Can you work these out from the model? Positions are in its coordinate system, mm. A direction names the side the tool comes from. Give positions to 0.01 mm unless a question says otherwise; leave off trailing zeros. Order: outer loops, then holes, each group sorted by start corner. A loop starts at its lowest first (then second) coordinate and runs counter-clockwise, first axis right, second up. Notation, with made-up numbers: M -7,-36.75 L 7,-36.75 A21 cw 7,-2.75 Z; hole C -2.5,-15 d3. An arc over 180 degrees is marked long. Write each question's results on one line, items separated by ' | '.
from build123d import *

# Parameters (mm, degrees)
SKETCH_1_R          = 10
EXTRUDE_1_DEPTH     = 20
SKETCH_2_R          = 5
EXTRUDE_2_DEPTH     = 5
SKETCH_4_R          = 5.5
SKETCH_4_R_2        = 5
EXTRUDE_3_DEPTH     = 1
SKETCH_5_R          = 1.65
CUT_EXTRUDE_1_DEPTH = 10
SKETCH_6_R          = 5
EXTRUDE_4_DEPTH     = 35.5
SKETCH_7_OUTSIDE_W  = 35.358
SKETCH_7_OUTSIDE_H  = 35.358
SKETCH_7_OUTSIDE_R  = 4
CUT_EXTRUDE_2_DEPTH = 16
SKETCH_8_R          = 1.65
CUT_EXTRUDE_3_DEPTH = 10
SKETCH_9_R          = 4
CUT_EXTRUDE_4_DEPTH = 0.8


with BuildPart() as part:
    # ｽｹｯﾁ1 → ﾎﾞｽ - 押し出し1 (new body)
    with BuildSketch(Plane.XY):
        Circle(SKETCH_1_R)
    extrude(amount=EXTRUDE_1_DEPTH)

    # ｽｹｯﾁ2 → ﾎﾞｽ - 押し出し2 (add)
    with BuildSketch(Plane.XY.offset(20)):
        Circle(SKETCH_2_R)
    extrude(amount=EXTRUDE_2_DEPTH)

    # ｽｹｯﾁ4 → ﾎﾞｽ - 押し出し3 (add)
    with BuildSketch(Plane.XY.offset(20)):
        Circle(SKETCH_4_R)
        Circle(SKETCH_4_R_2, mode=Mode.SUBTRACT)
    extrude(amount=EXTRUDE_3_DEPTH)

    # ｽｹｯﾁ5 → ｶｯﾄ - 押し出し1 (cut)
    with BuildSketch(Plane(origin=(0, 0, 0), x_dir=(-1, 0, 0), z_dir=(0, 0, -1))):
        with Locations((0, 6)):
            Circle(SKETCH_5_R)
        with Locations(Location((0, -6, 0), (0, 0, 180))):
            Circle(SKETCH_5_R)
    extrude(amount=-CUT_EXTRUDE_1_DEPTH, mode=Mode.SUBTRACT)

    # ｽｹｯﾁ6 → ﾎﾞｽ - 押し出し4 (add)
    with BuildSketch(Plane.XY.offset(25)):
        Circle(SKETCH_6_R)
    extrude(amount=EXTRUDE_4_DEPTH)

    # ｽｹｯﾁ7 outside → ｶｯﾄ - 押し出し2 (cut)
    with BuildSketch(Plane.XY.offset(60.5)):
        Rectangle(SKETCH_7_OUTSIDE_W, SKETCH_7_OUTSIDE_H)
        Circle(SKETCH_7_OUTSIDE_R, mode=Mode.SUBTRACT)
    extrude(amount=-CUT_EXTRUDE_2_DEPTH, mode=Mode.SUBTRACT)

    # ｽｹｯﾁ8 → ｶｯﾄ - 押し出し3 (cut)
    with BuildSketch(Plane.XY.offset(60.5)):
        Circle(SKETCH_8_R)
    extrude(amount=-CUT_EXTRUDE_3_DEPTH, mode=Mode.SUBTRACT)

    # ｽｹｯﾁ9 → ｶｯﾄ - 押し出し4 (cut)
    with BuildSketch(Plane.XY.offset(60.5)):
        Circle(SKETCH_9_R)
    extrude(amount=-CUT_EXTRUDE_4_DEPTH, mode=Mode.SUBTRACT)


solid = part.part
(1) Imagine slicing it at B-B, the plane y = 0. Write out the boundary of the cut face in (x, z).
Data:
outline: M -10,0 L 10,0 L 10,20 L 5.5,20 L 5.5,21 L 5,21 L 5,44.5 L 4,44.5 L 4,59.7 L 1.65,59.7 L 1.65,50.5 L -1.65,50.5 L -1.65,59.7 L -4,59.7 L -4,44.5 L -5,44.5 L -5,21 L -5.5,21 L -5.5,20 L -10,20 Z
(2) I need wall thicknesses on L1, parallel to Y at x = 0, z = 3.5; L2, parallel to Y at x = 0, z = 53.5; L3, parallel to Z at x = 7, y = -4. Which ranges of each line are inside material? Lowest first, please. Write a range as from..to.
Data:
L1: y = -10..-7.65, -4.35..4.35, 7.65..10 | L2: y = -4..-1.65, 1.65..4 | L3: z = 0..20
(3) Imagine slicing it at C-C, the plane z = 48. Write out the boundary of the cut face in (x, y).
Data:
outline: C 0,0 d8
(4) Will these pins go through, and if not, where does the flat tip stop? P1, Ø4, axis at x = 4, z = 21.5, coming from the +Y side (3 decimals); P2, Ø12, axis at x = -3, z = 44.5, coming from the -Y side; P3, Ø10, axis at y = -7.5, z = 24, coming from the +X side.
Data:
P1: stops at y = 9.635 | P2: stops at y = -5 | P3: stops at x = 8.93
(5) We'd pull the mould along X, two halves only. Please class faces 4 (the face through (0, 0, 50.5)), 5 (the face through (-1.19, -5.37, 20.49)), 6 (the face through (2, 0, 59.7)): +X half, -X half, draft (parallel to the pull), parting line (faces both ways), or undercut.
Data:
face 4: undercut | face 5: parting line | face 6: draft
(6) For faces 1 (the face through (0, 6, 10)), 2 (the face through (-2.17, -9.76, 9.86)), 3 (the face through (4, -4, 20)), which set-ups out of +Z, -Z, +X, -X, +Y, -Y let a thin tool reach every point of the face, with its end or its side?
Data:
face 1: -Z | face 2: +Z, -Z | face 3: +Z
(7) Imagine slicing it at D-D, the plane z = 12. Write out the boundary of the cut face in (x, y).
Data:
outline: C 0,0 d20
(8) Imagine slicing it at A-A, the plane x = 0. Write out the boundary of the cut face in (y, z), plus the area to 3 significant figures.
Data:
outline: M -10,0 L -7.65,0 L -7.65,10 L -4.35,10 L -4.35,0 L 4.35,0 L 4.35,10 L 7.65,10 L 7.65,0 L 10,0 L 10,20 L 5.5,20 L 5.5,21 L 5,21 L 5,44.5 L 4,44.5 L 4,59.7 L 1.65,59.7 L 1.65,50.5 L -1.65,50.5 L -1.65,59.7 L -4,59.7 L -4,44.5 L -5,44.5 L -5,21 L -5.5,21 L -5.5,20 L -10,20 Z | area: 671 mm2
